Study the drawing (mm; zero at the part's minimum x, y, z) and answer. Coordinates: 2 decimals unless noted, no trailing zeros. Loops run counter-clockwise (first coordinate to the right, second up) from the corner with the lowest first, then second, coordinate; pieces in that order, holes last. Notation, with made-up numbers: (70.25, -30.75) -> (88.25, -30.75) arc R22 cw to (88.25, -7.75) -> close; hole circle Ø8 at (75.5, -27.75). An arc over 180 degrees is marked (long way). Answer as CSV lines item,"result".
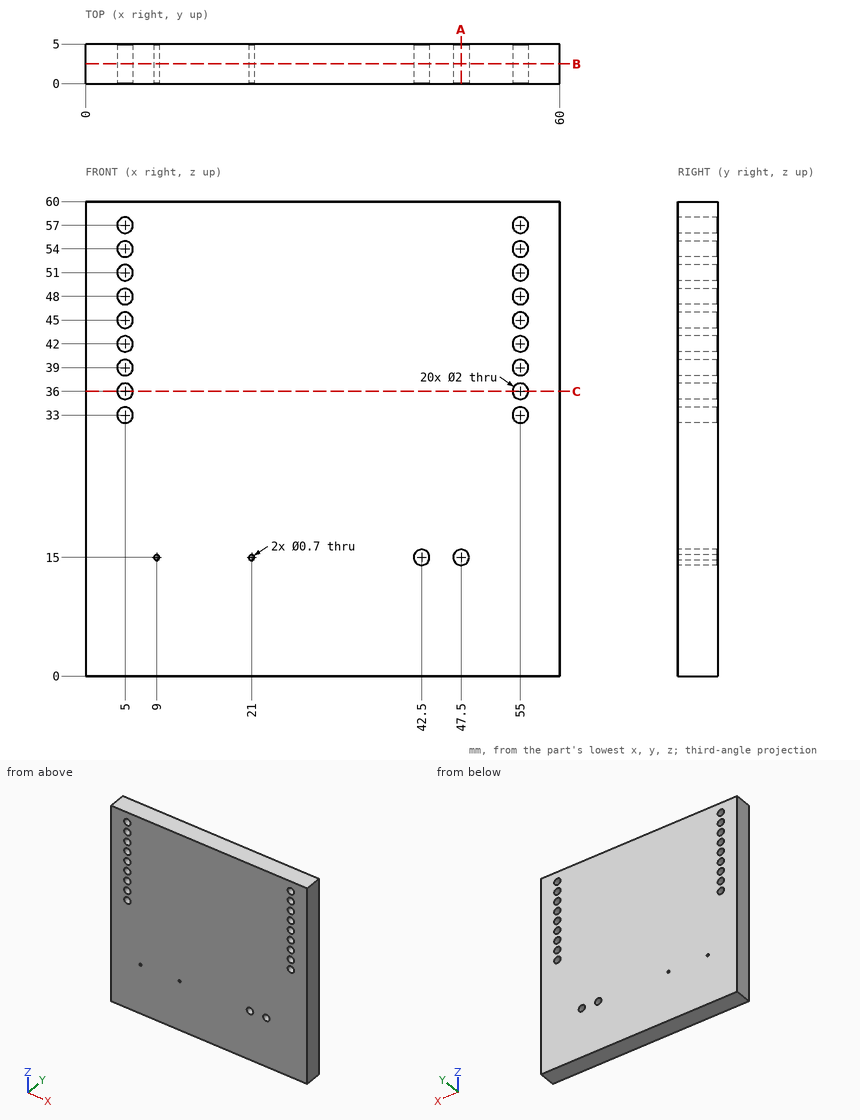
Q1. A cutting plane is placed at C-C, the plane z = 36. Write down the section's boundary in (x, y), and give its area (3 significant figures).
Results:
outline,"(0, 0) -> (4, 0) -> (4, 5) -> (0, 5) -> close; (6, 0) -> (54, 0) -> (54, 5) -> (6, 5) -> close; (56, 0) -> (60, 0) -> (60, 5) -> (56, 5) -> close"
area,"280 mm²"
Q2. A cutting plane is placed at A-A, the plane x = 47.5. Write down the section's boundary in (y, z).
Results:
outline,"(0, 0) -> (5, 0) -> (5, 14) -> (0, 14) -> close; (0, 16) -> (5, 16) -> (5, 60) -> (0, 60) -> close"
Q3. A cutting plane is placed at B-B, the plane y = 2.5. Give the number of separate pieces and of enclosed holes in the cut face, and give its area (3 significant figures).
Results:
separate pieces,"1"
enclosed holes,"22"
area,"3,540 mm²"
Q4. Find the intervals of material crossed by probe 1 along X at (y, z) = (1.65, 45); probe 2 along X at (y, z) = (1.45, 15); probe 3 along Z at (x, y) = (47.5, 2.1), in increasing order. Write a range as [from, to].
Results:
probe 1,"x = [0, 4], [6, 54], [56, 60]"
probe 2,"x = [0, 8.65], [9.35, 20.65], [21.35, 41.5], [43.5, 46.5], [48.5, 60]"
probe 3,"z = [0, 14], [16, 60]"
Q5. Given pin 1 Ø1.8 at (x, z) = (42.5, 15) entering from +Y, flat-ended and moving along its own axis, determine where the tip first touches the part or whether it passes through.
Results:
pin 1,"passes through"
